Read the model definition and answer for the solid it produces. Units are mm, in the model's axes. Face numbers are marked on the shaded views. A direction names the side the tool comes from. Coordinates: 2 decimals unless noted, no trailing zeros. Loops run counter-clockwise (first coordinate to the right, second up) from the corner with the lowest first, then second, coordinate; pieces in that order, holes last. Notation, with made-up numbers: (5, 66.5) -> (55, 66.5) arc R34 cw to (55, 105.5) -> close; hole circle Ø6 at (-0.75, 56.5). An arc over 180 degrees is marked (long way). Answer as CSV lines item,"result".
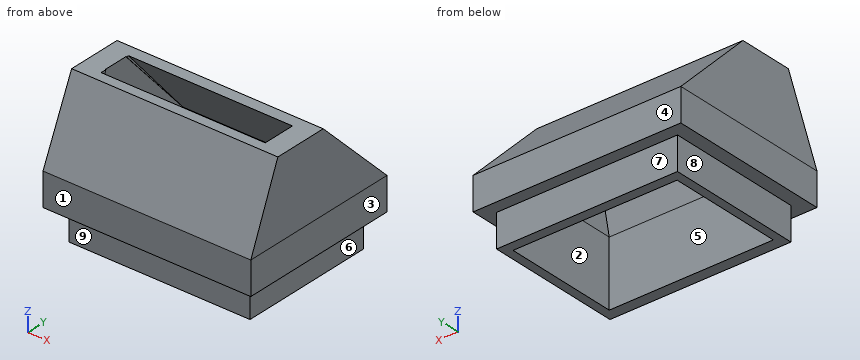
Autodesk Fusion 360 part; units mm, degrees
sketch "Sketch1" plane through (0, 0, 0) normal (0, 0, 1) x (1, 0, 0)
  line L0 (-8.7725, 5.8867) -> (7.7775, 5.8867)
  line L1 (7.7775, 5.8867) -> (7.7775, -6.6133)
  line L2 (7.7775, -6.6133) -> (-8.7725, -6.6133)
  line L3 (-8.7725, -6.6133) -> (-8.7725, 5.8867)
  line L4 (-8, 5) -> (6.9982, 5)
  line L5 (6.9982, 5) -> (6.9982, -5.595)
  line L6 (6.9982, -5.595) -> (-8, -5.595)
  line L7 (-8, -5.595) -> (-8, 5)
  dimension "d1" = 16.55
  dimension "d2" = 12.5
extrude "Extrude1" add sketch "Sketch1" along normal blind 3
sketch "Sketch2" plane through (0, 0, 3) normal (0, 0, 1) x (-1, 0, 0)
  line L0 (-6.9982, 5.595) -> (8, 5.595)
  line L1 (8, 5.595) -> (8, -5)
  line L2 (8, -5) -> (-6.9982, -5)
  line L3 (-6.9982, -5) -> (-6.9982, 5.595)
  line L4 (8.7725, 6.6133) -> (-7.7775, 6.6133)
  line L5 (-7.7775, 6.6133) -> (-7.7775, -5.8867)
  line L6 (-7.7775, -5.8867) -> (8.7725, -5.8867)
  line L7 (8.7725, -5.8867) -> (8.7725, 6.6133)
  line L8 (10, -7) -> (-9, -7)
  line L9 (-9, -7) -> (-9, 8)
  line L10 (-9, 8) -> (10, 8)
  line L11 (10, 8) -> (10, -7)
extrude "Extrude2" add sketch "Sketch2" along normal blind 3 contours L4 L5 L6 L7 | L8 L9 L10 L11
ref_plane "WorkPlane1" through (-0.5, -0.5, 13) normal (0, 0, 1) x (1, 0, 0)
sketch "Sketch4" plane through (-0.5, -0.5, 13) normal (0, 0, 1) x (1, 0, 0)
  line L0 (-9.442, -4.4154) -> (9.4117, -4.4154)
  line L1 (9.4117, -4.4154) -> (9.4117, 0.5846)
  line L2 (9.4117, 0.5846) -> (-9.442, 0.5846)
  line L3 (-9.442, 0.5846) -> (-9.442, -4.4154)
  line L4 (-7.5524, -2.9878) -> (7.4802, -2.9878)
  line L5 (7.4802, -2.9878) -> (7.4802, -0.7203)
  line L6 (7.4802, -0.7203) -> (-7.5524, -0.7203)
  line L7 (-7.5524, -0.7203) -> (-7.5524, -2.9878)
  dimension "d8" = 5
sketch "Sketch5" plane through (0, 0, 6) normal (0, 0, 1) x (-1, 0, 0)
  line L0 (8, -5) -> (-6.9982, -5)
  line L1 (-6.9982, -5) -> (-6.9982, 5.595)
  line L2 (-6.9982, 5.595) -> (8, 5.595)
  line L3 (8, 5.595) -> (8, -5)
  line L4 (10, 8) -> (-9, 8)
  line L5 (-9, 8) -> (-9, -7)
  line L6 (-9, -7) -> (10, -7)
  line L7 (10, -7) -> (10, 8)
  line L8 (10, -7) -> (-9, -7)
  line L9 (-9, -7) -> (-9, 8)
  line L10 (-9, 8) -> (10, 8)
  line L11 (10, 8) -> (10, -7)
loft "Loft1" add profiles "Sketch5", "Sketch4" section 1 section 2
sketch "Sketch6" plane through (0, 0, 13) normal (0, 0, 1) x (-1, 0, 0)
  line L0 (9.942, 4.9154) -> (-8.9117, 4.9154)
  line L1 (-8.9117, 4.9154) -> (-8.9117, -0.0846)
  line L2 (-8.9117, -0.0846) -> (9.942, -0.0846)
  line L3 (9.942, -0.0846) -> (9.942, 4.9154)
  line L4 (8, 1) -> (-7, 1)
  line L5 (-7, 1) -> (-7, 4)
  line L6 (-7, 4) -> (8, 4)
  line L7 (8, 4) -> (8, 1)
sketch "Sketch7" plane through (0, 0, 6) normal (0, 0, -1) x (1, 0, 0)
  line L0 (6.9982, -5) -> (6.9982, 5.595)
  line L1 (6.9982, 5.595) -> (-8, 5.595)
  line L2 (-8, 5.595) -> (-8, -5)
  line L3 (-8, -5) -> (6.9982, -5)
  line L4 (-8, 5.595) -> (6.9982, 5.595)
  line L5 (6.9982, 5.595) -> (6.9982, -5)
  line L6 (6.9982, -5) -> (-8, -5)
  line L7 (-8, -5) -> (-8, 5.595)
loft "Loft2" cut profiles "Sketch7", "Sketch6" section 1 section 2 contours L4 L5 L6 L7
Q1. A cutting plane is placed at A-A, the plane z = 4. Write down the section's boundary in (x, y) (3 decimals), and give its area (3 significant figures).
Results:
outline,"(-10, -8) -> (9, -8) -> (9, 7) -> (-10, 7) -> close; hole (-8, -5.595) -> (6.998, -5.595) -> (6.998, 5) -> (-8, 5) -> close"
area,"126 mm²"
Q2. Given pin 1 Ø0.9 at (x, z) = (-2, 1.5) entering from +Y; pin 2 Ø3 at (x, z) = (5.5, 9) entering from -Y; pin 3 Ø4 at (x, z) = (-3, 10.5) entering from -Y, each flat-ended and moving along its own axis, determine where each tip first touches the part or whether it passes through.
Results:
pin 1,"stops at y = 5.89"
pin 2,"stops at y = -7.34"
pin 3,"stops at y = -6.9"
Q3. For the marked faces 5, 6, 7, 8 and 9, determine the directions among +Z, -Z, +X, -X, +Y, -Y from which every point of the face is accessible in a straight line to the end or side of a thin tool.
Results:
face 5,"-Z"
face 6,"-Z, +X, +Y, -Y"
face 7,"-Z, +X, -X, +Y"
face 8,"-Z, -X, +Y, -Y"
face 9,"-Z, +X, -X, -Y"
Q4. Find the intervals of material crossed by probe 1 along X at (y, z) = (2.25, 6.25); probe 2 along Y at (x, z) = (2.5, 5.5) (3 decimals); probe 3 along Y at (x, z) = (-6.25, 8.5), in increasing order. Write a range as [from, to].
Results:
probe 1,"x = [-10, -8], [7, 9]"
probe 2,"y = [-8, -5.595], [5, 7]"
probe 3,"y = [-6.9, -5.03], [2.86, 4.53]"
Q5. For a pull along Y with two mould halves and no side action, classify the marked faces 1, 2, 3 and 4 as pulls with the +Y half, pulls with the -Y half, needs draft (parallel to the pull), parting line crosses it, or undercut.
Results:
face 1,"pulls with the -Y half"
face 2,"undercut"
face 3,"needs draft"
face 4,"pulls with the +Y half"
